Here's the drawing with two shaded views (mm, measured from the low corner). I have some questions. A direction names the side the tool comes from. Coordinates: 2 decimals unless noted, no trailing zeros. Order: outer loops, then holes, each group sorted by start corner. A loop starts at its lowest first (then second) coordinate and runs counter-clockwise, first axis right, second up. Notation, with made-up numbers: (-13, 74.5) -> (25, 74.5) arc R28 ccw to (25, 109.5) -> close; hole circle Ø3 at (49, -15). An arc over 180 degrees is marked (long way). Return JSON: item names as keys, results as strings. Group by question number.
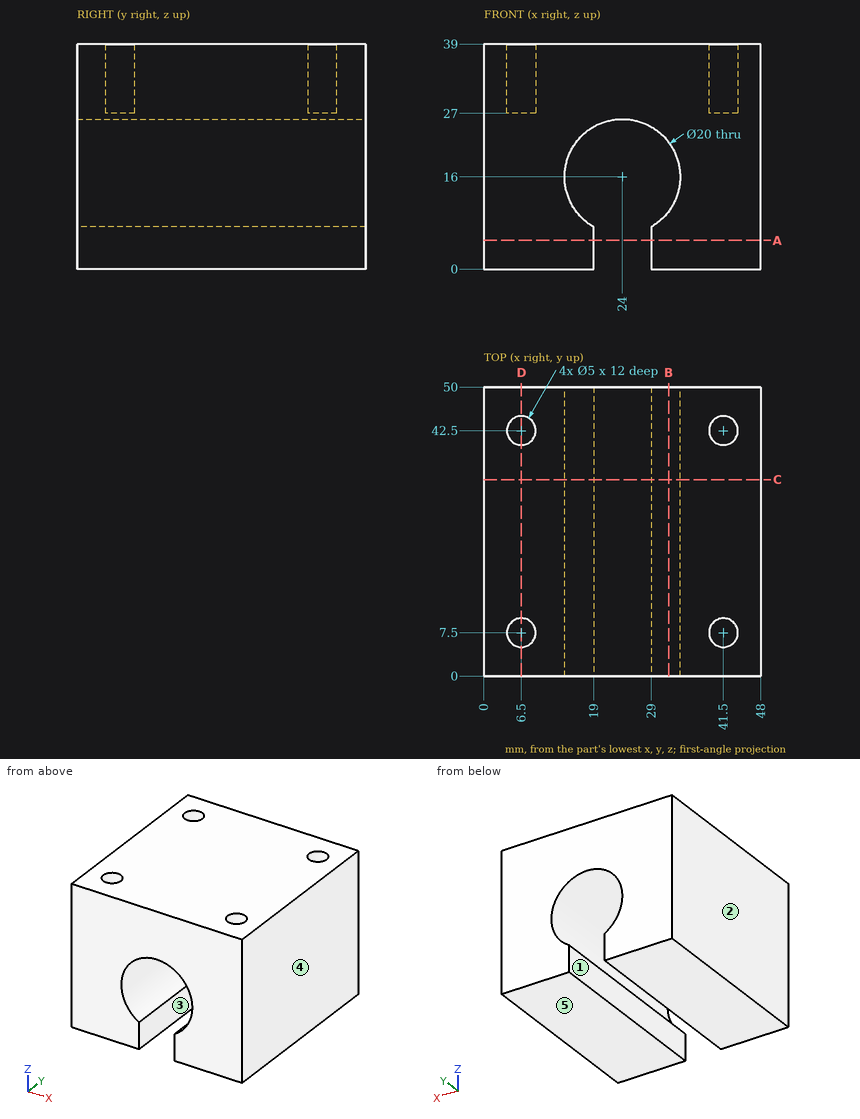
Q1. I'm going to push a flat-ended pin straight in: pin 1 Ø2.5 at (x, y) = (41.5, 42.5) entering from +Z. Where does the tip first touch, or does it pass through?
Q2. I want a section at B-B on x = 32. Please give me the cut outline in (y, z), and give its area (3 significant figures).
Q3. On a 3-axis mill with a long thin cutter (end or side, diameter ignored), from which of +Z, -Z, +X, -X, +Y, -Y can I reach the whole of each face in a straight line? I mean the marked faces 1 and 2. Say none if no direction works.
Q4. I need wall thicknesses on line 1 along Y through (x, z) = (6.5, 31.25); line 2 along X through (y, z) = (16, 6.5); line 3 along Y through (x, z) = (43, 32). Which ranges of each line are inside material? Lowest first, please. Write a range as from..to.
Q5. I want a section at A-A on z = 5. Please give me the cut outline in (x, y), and give its area (3 significant figures).
Q6. I want a section at C-C on y = 34. Please give me the cut outline in (x, z), and give its area (3 significant figures).
Q7. I want a section at D-D on x = 6.5. Please give me the cut outline in (y, z).
Q8. We'd pull the mould along X, two halves only. Please class the marked faces 3, 4 and 5: pulls with the +X half, pulls with the -X half, needs draft (parallel to the pull), parting line crosses it, or undercut.
Response values:
{
 "1": {"pin 1": "stops at z = 27"},
 "2": {"outline": "(0, 0) -> (50, 0) -> (50, 10) -> (0, 10) -> close; (0, 22) -> (50, 22) -> (50, 39) -> (0, 39) -> close", "area": "1,350 mm²"},
 "3": {"face 1": "-Z, +Y, -Y", "face 2": "+Z, -Z, -X, +Y, -Y"},
 "4": {"line 1": "y = 0..5, 10..40, 45..50", "line 2": "x = 0..19, 29..48", "line 3": "y = 0..5.5, 9.5..40.5, 44.5..50"},
 "5": {"outline": "(0, 0) -> (19, 0) -> (19, 50) -> (0, 50) -> close; (29, 0) -> (48, 0) -> (48, 50) -> (29, 50) -> close", "area": "1,900 mm²"},
 "6": {"outline": "(0, 0) -> (19, 0) -> (19, 7.34) arc R10 cw (long way) to (29, 7.34) -> (29, 0) -> (48, 0) -> (48, 39) -> (0, 39) -> close", "area": "1,490 mm²"},
 "7": {"outline": "(0, 0) -> (50, 0) -> (50, 39) -> (45, 39) -> (45, 27) -> (40, 27) -> (40, 39) -> (10, 39) -> (10, 27) -> (5, 27) -> (5, 39) -> (0, 39) -> close"},
 "8": {"face 3": "undercut", "face 4": "pulls with the +X half", "face 5": "needs draft"}
}
